Model file for the job. Use its own axes, mm. A direction names the side the tool comes from. Give positions to 0.01 mm unless a question says otherwise; leave off trailing zeros. Order: outer loops, then holes, each group sorted by start corner. A loop starts at its lowest first (then second) coordinate and runs counter-clockwise, first axis right, second up. Notation, with made-up numbers: (87.5, 57.25) - (145.5, 57.25) arc R34 ccw to (145.5, 89.25) - close; hole circle Ø10 at (35.5, 75). An arc over 180 degrees is marked (long way). Return JSON: item names as keys, results as strings. Group by question number.
from build123d import *

# Parameters (mm, degrees)
BOSS_EXTRUDE1_DEPTH = 3.175
SKETCH3_W           = 12.7
SKETCH3_H           = 6.35
CUT_EXTRUDE1_DEPTH  = 1.778
BOSS_EXTRUDE2_DEPTH = 3.175


with BuildPart() as part:
    # Sketch2 → Boss-Extrude1 (new body)
    with BuildSketch(Plane.XY):
        Polygon((0, 0), (12.7, 0), (12.7, 6.35), (17.145, 6.35), (17.145, 21.59), (-6.35, 21.59), (-64.77, 80.01), (-67.945, 80.01), (-67.945, 16.51), (-48.895, 16.51), (-48.895, 12.7), (-36.195, 12.7), (-36.195, 16.51), (-4.445, 16.51), (-4.445, 6.35), (0, 6.35), align=None)
        Polygon((-64.77, 71.029743879), (-64.77, 23.83506403), (-41.172660076, 47.432403955), align=None, mode=Mode.SUBTRACT)
        Polygon((-62.52493597, 21.59), (-15.330256121, 21.59), (-38.927596045, 45.187339924), align=None, mode=Mode.SUBTRACT)
    extrude(amount=BOSS_EXTRUDE1_DEPTH)

    # Sketch3 → Cut-Extrude1 (cut)
    with BuildSketch(Plane(origin=(0, 0, 0), x_dir=(-1, 0, 0), z_dir=(0, 0, -1))):
        with Locations((-6.35, 3.175)):
            Rectangle(SKETCH3_W, SKETCH3_H)
    extrude(amount=-CUT_EXTRUDE1_DEPTH, mode=Mode.SUBTRACT)

    # Sketch4 → Boss-Extrude2 (add)
    with BuildSketch(Plane(origin=(0, 0, 0), x_dir=(-1, 0, 0), z_dir=(0, 0, -1))):
        Polygon((15.330256121, 21.59), (64.77, 71.029743879), (62.929047495, 72.870696384), (13.489303616, 23.430952505), align=None)
        Polygon((10.840128061, 26.080128061), (12.681080565, 24.239175556), (62.120824444, 73.678919435), (60.279871939, 75.519871939), align=None)
    extrude(amount=BOSS_EXTRUDE2_DEPTH)


solid = part.part
(1) Slice it at C-C (x = -22). Give the cut face in (y, z) (3 decimals), and give its area (3 significant figures).
(2) Pull direction Y, two halves, no side cores. Call faces 4 (the face through (-38.56, 48.5, -1.57)), 5 (the face through (-36, 50, -3.175)), 6 (the face through (-66, 80.01, 2)): released by +Y, released by -Y, zero draft, split by the parting line, or undercut.
(3) Drop flat-ended pins along their axis: pin 1 Ø1.5 at (y, z) = (40, 2) entering from +X; pin 2 Ø5 at (x, y) = (9.5, 4) entering from -Z; pin 3 Ø1.5 at (y, z) = (2, 2.5) entering from +X. Give the stop position or say it passes through.
(4) Drill centre lines: L1, parallel to X at y = 44, z = 1.5 (3 decimals); L2, parallel to Z at x = -12.5, y = 21 (3 decimals); L3, parallel to X at y = 51, z = 1.25 (3 decimals). Where is each one in solid material? Low to high.
(5) Slice it at D-D (y = 37). Give the cut face in (x, z) (3 decimals), and give its area (3 significant figures).
(6) Slice it at B-B (z = -2). Give the cut face in (x, y).
(7) 3-axis set-ups, long thin cutter, end or side, ignore diameter. For faces 1 (the face through (-36.195, 15, 2)), 2 (the face through (-53.137, 35.469, 1.565)), 3 (the face through (-59, 16.51, 2)): which of +Z, -Z, +X, -X, +Y, -Y reach the whole face in a straight line?
(8) Slice it at A-A (y = 15). Give the cut face in (x, z) (3 decimals).
Result set:
{
 "1": {"outline": "(16.51, 0) - (21.59, 0) - (21.59, 3.175) - (16.51, 3.175) - close; (28.26, -3.175) - (31.942, -3.175) - (31.942, 0) - (33.558, 0) - (33.558, -3.175) - (37.24, -3.175) - (37.24, 3.175) - (28.26, 3.175) - close", "area": "68.0 mm²"},
 "2": {"face 4": "undercut", "face 5": "zero draft", "face 6": "released by +Y"},
 "3": {"pin 1": "stops at x = -24.01", "pin 2": "stops at z = 0", "pin 3": "stops at x = 12.7"},
 "4": {"L1": "x = -67.945 to -64.77, -44.605 to -40.115, -37.74 to -28.76", "L2": "z = 0 to 3.175", "L3": "x = -67.945 to -64.77, -44.74 to -35.76"},
 "5": {"outline": "(-67.945, 0) - (-64.77, 0) - (-64.77, 3.175) - (-67.945, 3.175) - close; (-51.605, 0) - (-47.115, 0) - (-47.115, 3.175) - (-51.605, 3.175) - close; (-30.74, -3.175) - (-27.058, -3.175) - (-27.058, 0) - (-25.442, 0) - (-25.442, -3.175) - (-21.76, -3.175) - (-21.76, 3.175) - (-30.74, 3.175) - close", "area": "76.2 mm²"},
 "6": {"outline": "(-64.77, 71.03) - (-15.33, 21.59) - (-13.49, 23.43) - (-62.93, 72.87) - close; (-62.12, 73.68) - (-12.68, 24.24) - (-10.84, 26.08) - (-60.28, 75.52) - close"},
 "7": {"face 1": "+Z, -Z, -Y", "face 2": "+Z, -Z", "face 3": "+Z, -Z, -X, -Y"},
 "8": {"outline": "(-48.895, 0) - (-36.195, 0) - (-36.195, 3.175) - (-48.895, 3.175) - close; (-4.445, 0) - (17.145, 0) - (17.145, 3.175) - (-4.445, 3.175) - close"}
}
